```python
from build123d import *

# Parameters (mm, degrees)
F0_W     = 203.2
F0_H     = 127
F1_DEPTH = 50.8
F2_R     = 15.875
F3_DEPTH = 50.801
F4_R     = 6.35


with BuildPart() as f1:
    # F0 (on Front) → F1 (new body)
    with BuildSketch(Plane.XZ):
        with Locations((101.6, 63.5)):
            Rectangle(F0_W, F0_H)
    extrude(amount=F1_DEPTH)

    # F2 (on face) → F3 (cut, through all)
    with BuildSketch(Plane.XZ.offset(50.8)):
        with Locations((203.2, 63.5)):
            Circle(F2_R)
    extrude(amount=-F3_DEPTH, mode=Mode.SUBTRACT)

    # F4
    f4_edges = [f1.edges().sort_by_distance(p)[0] for p in [
        (203.2, -25.4, 127),
        (203.2, -25.4, 0),
        (0, -25.4, 127),
        (0, -25.4, 0),
    ]]
    fillet(f4_edges, radius=F4_R)


solid = f1.part
```
CAD build for the part. Positions are in the model's coordinates, mm. Coordinates: 2 decimals unless noted, no trailing zeros. Write each loop counter-clockwise with the first axis right and the second up, starting at its lowest first coordinate (ties: lowest second). Pieces come first, ordered by that corner, then holes.
(1) Flat gauge pins, fed straight in: pin 1 (1.5 mm diameter, centred on y = -42.5, z = 63, fed in from +X); pin 2 (1.5 mm diameter, centred on y = -35, z = 74, fed in from +X). Where does each tip first touch, or does it go through?
(2) Cut at A-A, the plane y = -27. List the corners of the cut face in (x, z) (3 decimals), and give its area (3 significant figures).
(3) Drill centre lines: probe 1 along Z at (x, y) = (189, -33); probe 2 along X at (y, z) = (-10, 5); probe 3 along X at (y, z) = (-14.5, 53). Where is each one in solid material? Low to high.
(4) Cut at B-B, the plane z = 63.5. List the corners of the cut face in (x, y) (3 decimals), and give its area (3 significant figures).
Geometry says:
1. pin 1: stops at x = 187.37
1. pin 2: stops at x = 192
2. outline: (0, 6.35) arc R6.35 ccw to (6.35, 0) - (196.85, 0) arc R6.35 ccw to (203.2, 6.35) - (203.2, 47.625) arc R15.875 cw to (203.2, 79.375) - (203.2, 120.65) arc R6.35 ccw to (196.85, 127) - (6.35, 127) arc R6.35 ccw to (0, 120.65) - close
2. area: 25,400 mm2
3. probe 1: z = 0 to 56.4, 70.6 to 127
3. probe 2: x = 0.15 to 203.05
3. probe 3: x = 0 to 191.29
4. outline: (0, -50.8) - (187.325, -50.8) - (187.325, 0) - (0, 0) - close
4. area: 9,520 mm2
